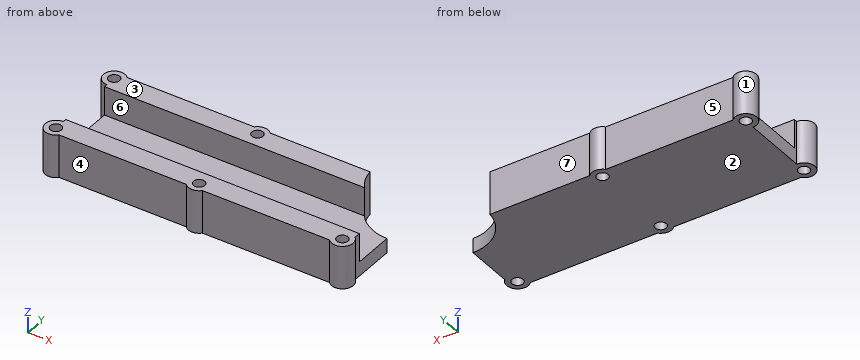
```python
from build123d import *

# Parameters (mm, degrees)
SKETCH1_R           = 2.4892
BOSS_EXTRUDE1_DEPTH = 19.05
SKETCH2_W           = 12.7
SKETCH2_H           = 25.4
CUT_EXTRUDE1_DEPTH  = 140.862263719


with BuildPart() as part:
    # Sketch1 → Boss-Extrude1 (new body)
    # profile 1 of 2: a face of its own
    with BuildSketch(Plane.XY):
        with BuildLine():
            ThreePointArc((-3.549757914, -3.175), (0, -4.7625), (3.549757914, -3.175))
            Line((3.549757914, -3.175), (59.950242086, -3.175))
            ThreePointArc((59.950242086, -3.175), (66.867596045, -3.367596045), (66.675, 3.549757914))
            Line((66.675, 3.549757914), (66.675, 24.4475))
            ThreePointArc((66.675, 24.4475), (54.014749706, 29.263015025), (47.755090017, 41.275))
            Line((47.755090017, 41.275), (3.549757914, 41.275))
            Line((3.549757914, 41.275), (-3.549757914, 41.275))
            Line((-3.549757914, 41.275), (-59.950242086, 41.275))
            ThreePointArc((-59.950242086, 41.275), (-67.8475478, 40.044282483), (-63.5, 33.3375))
            Line((-63.5, 33.3375), (-63.5, 4.7625))
            ThreePointArc((-63.5, 4.7625), (-67.8475478, -1.944282483), (-59.950242086, -3.175))
            Line((-59.950242086, -3.175), (-3.549757914, -3.175))
        make_face()
        with Locations(Location((-63.5, 0, 0), (0, 0, 180))):
            Circle(SKETCH1_R, mode=Mode.SUBTRACT)
        with Locations(Location((0, 0, 0), (0, 0, 180))):
            Circle(SKETCH1_R, mode=Mode.SUBTRACT)
        with Locations(Location((63.5, 0, 0), (0, 0, 180))):
            Circle(SKETCH1_R, mode=Mode.SUBTRACT)
        with Locations(Location((-63.5, 38.1, 0), (0, 0, 180))):
            Circle(SKETCH1_R, mode=Mode.SUBTRACT)
        with Locations(Location((0, 38.1, 0), (0, 0, 180))):
            Circle(SKETCH1_R, mode=Mode.SUBTRACT)
    # profile 2 of 2: a face of its own
    with BuildSketch(Plane.XY):
        with BuildLine():
            Line((-3.549757914, 41.275), (3.549757914, 41.275))
            ThreePointArc((3.549757914, 41.275), (0, 42.8625), (-3.549757914, 41.275))
        make_face()
    extrude(amount=BOSS_EXTRUDE1_DEPTH)

    # Sketch2 → Cut-Extrude1 (cut, through all)
    with BuildSketch(Plane.ZY.offset(63.5)):
        with Locations((6.35, 19.05)):
            Rectangle(SKETCH2_W, SKETCH2_H)
    extrude(amount=-CUT_EXTRUDE1_DEPTH, mode=Mode.SUBTRACT)


with BuildPart() as body_2:
    # Mirror1: mirrored copy
    add(part.part.mirror(Plane.XY.offset(19.05)))


solid = body_2.part
```
Work out the finished part from the listing and answer in its coordinate system (mm). Face numbers are marked on the shaded views. A direction names the side the tool comes from. Round coordinates to 2 decimals unless told otherwise and drop trailing zeros. Loops run counter-clockwise (first coordinate to the right, second up) from the corner with the lowest first, then second, coordinate; pieces in that order, holes last. Notation, with made-up numbers: (62.5, -30) -> (77.5, -30) arc R16 ccw to (77.5, -19) -> close; hole circle Ø1 at (-28.5, 7). An arc over 180 degrees is marked (long way). Write each question's results on one line, items separated by ' | '. Start each with the question number.
1. Section C-C (x = 0) is taken. Determine the outline of the cut face in (y, z).
2. Given pin 1 Ø5.5 at (y, z) = (17.5, 26) entering from +X (3 decimals); pin 2 Ø10 at (x, z) = (46, 26.5) entering from +Y (3 decimals); pin 3 Ø7.5 at (x, y) = (-6.5, 14) entering from +Z, each flat-ended and moving along its own axis, determine where each tip first touches the part or whether it passes through.
3. Section A-A (z = 35) is taken. State how many separate pieces and enclosed holes the cut face has, plus the area to 3 significant figures.
4. Section B-B (y = 0) is taken. Determine the outline of the cut face in (x, z), plus the area to 3 significant figures.
5. Find the intervals of material crossed by probe 1 along Y at (x, z) = (0, 33.25); probe 2 along Y at (x, z) = (-36.5, 30.25) (3 decimals); probe 3 along Z at (x, y) = (-0.5, 25.5), in increasing order. Write a range as from..to.
6. A tool of negligible diameter and unlimited length cuts with its end or side. For the marked faces 4, 5, 6 and 7, from which of +Z, -Z, +X, -X, +Y, -Y can it reach the whole face along a straight path? Write none if from no direction.
7. For a pull along Z with two mould halves and no side action, classify the marked faces 1, 2 and 3 as +Z half, -Z half, draft (parallel to the pull), parting line (faces both ways), or undercut.
Evaluation:
1) outline: (-4.76, 19.05) -> (-2.49, 19.05) -> (-2.49, 38.1) -> (-4.76, 38.1) -> close; (2.49, 19.05) -> (35.61, 19.05) -> (35.61, 38.1) -> (31.75, 38.1) -> (31.75, 25.4) -> (6.35, 25.4) -> (6.35, 38.1) -> (2.49, 38.1) -> close; (40.59, 19.05) -> (42.86, 19.05) -> (42.86, 38.1) -> (40.59, 38.1) -> close
2) pin 1: stops at x = 66.675 | pin 2: stops at y = 41.275 | pin 3: stops at z = 25.4
3) separate pieces: 2 | enclosed holes: 5 | area: 2,330 mm2
4) outline: (-68.26, 19.05) -> (-65.99, 19.05) -> (-65.99, 38.1) -> (-68.26, 38.1) -> close; (-61.01, 19.05) -> (-2.49, 19.05) -> (-2.49, 38.1) -> (-61.01, 38.1) -> close; (2.49, 19.05) -> (61.01, 19.05) -> (61.01, 38.1) -> (2.49, 38.1) -> close; (65.99, 19.05) -> (68.26, 19.05) -> (68.26, 38.1) -> (65.99, 38.1) -> close | area: 2,320 mm2
5) probe 1: y = -4.76..-2.49, 2.49..6.35, 31.75..35.61, 40.59..42.86 | probe 2: y = -3.175..6.35, 31.75..41.275 | probe 3: z = 19.05..25.4
6) face 4: +Z, -Z, -Y | face 5: +Z, -Z, +Y | face 6: +Z, +X, -X | face 7: +Z, -Z, +X, +Y
7) face 1: draft | face 2: -Z half | face 3: +Z half
